```python
from build123d import *

# Parameters (mm, degrees)
SKETCH2_R                = 4
SKETCH2_R_2              = 3.5
BOSS_EXTRUDE1_DEPTH      = 10
BOSS_EXTRUDE2_REACH      = 15.601
BOSS_EXTRUDE2_END_RADIUS = 4
SKETCH3_R                = 3
SKETCH3_R_2              = 2.5
SKETCH4_R                = 4
BOSS_EXTRUDE3_DEPTH      = 0.5
FILLET2_R                = 0.5


with BuildPart() as part:
    # Sketch2 → Boss-Extrude1 (new body)
    with BuildSketch(Plane.XY.offset(8)):
        Circle(SKETCH2_R)
        Circle(SKETCH2_R_2, mode=Mode.SUBTRACT)
    extrude(amount=BOSS_EXTRUDE1_DEPTH)


with BuildPart() as body_2:
    # Mirror2: mirrored copy
    add(part.part.mirror(Plane.XY.offset(8)))

    # Boss-Extrude2: up to this cylinder (the profile starts outside it)
    boss_extrude2_end = Plane(origin=(0, 0, 5.872578), z_dir=(0, 0, 1)) * Cylinder(BOSS_EXTRUDE2_END_RADIUS, 40.202, mode=Mode.PRIVATE)
    # Sketch3 → Boss-Extrude2 (add, up to the surface)
    with BuildSketch(Plane(origin=(8, 0, 3), x_dir=(0, 0, -1), z_dir=(1, 0, 0)), mode=Mode.PRIVATE) as boss_extrude2_sk1:
        with Locations((0.042568871, 0)):
            Circle(SKETCH3_R)
        with Locations((0.042568871, 0)):
            Circle(SKETCH3_R_2, mode=Mode.SUBTRACT)
    boss_extrude2_tool1 = extrude(boss_extrude2_sk1.sketch, amount=-BOSS_EXTRUDE2_REACH, mode=Mode.PRIVATE) - boss_extrude2_end
    add(boss_extrude2_tool1.solids().sort_by_distance((8, 0, 5.872578))[0])

    # Sketch4 → Boss-Extrude3 (add)
    with BuildSketch(Plane(origin=(0, 0, -2), x_dir=(-1, 0, 0), z_dir=(0, 0, -1))):
        Circle(SKETCH4_R)
    extrude(amount=BOSS_EXTRUDE3_DEPTH)

    # Fillet2
    fillet2_edges = [body_2.edges().sort_by_distance(p)[0] for p in [
        (4, 0, -2.5),
    ]]
    fillet(fillet2_edges, radius=FILLET2_R - 0.0001)  # a hair under: the kernel refuses the full size


solid = body_2.part
```
Verification items for the finished model (mm, model axes). A direction names the side the tool comes from. Round coordinates to 2 decimals unless told otherwise and drop trailing zeros. Order: outer loops, then holes, each group sorted by start corner. A loop starts at its lowest first (then second) coordinate and runs counter-clockwise, first axis right, second up. Notation, with made-up numbers: (31, 11) -> (60, 11) arc R27 cw to (60, 30) -> close; hole circle Ø6 at (-28, 83.25). An arc over 180 degrees is marked (long way). Put each result on its own line as item: value. Start each with the question number.
(1) Section check D-D (x = 5.5). Enter the section's corners in (y, z), then the cut area to 3 significant figures.
(2) Draft check along Z on faces 4 (the face through (4, 0, 3)), 5 (the face through (8, 2, 1)), 6 (the face through (0, 0, -2)). Enter one of: +Z half, -Z half, draft (parallel to the pull), parting line (faces both ways), or undercut.
(3) Material ranges on line 1 along Y through (x, z) = (0, -0.5); line 2 along Z through (x, y) = (1, -1.25); line 3 along X through (y, z) = (2.5, 4.25), recorded low to high.
(4) Depth check by flat-ended pin: pin 1 Ø2 at (x, y) = (-1, -1) entering from +Z; pin 2 Ø3 at (y, z) = (-2.5, 0.5) entering from -X; pin 3 Ø1.5 at (x, z) = (2, 6) entering from -Y. Enter the tip coordinate at first touch or a pass-through.
(5) Section check C-C (z = 0.75). Enter the section's corners in (x, y), then the cut area to 3 significant figures.
(6) Section check B-B (y = 0). Enter the section's corners in (x, z), then the cut area to 3 significant figures.
(7) Tool access check on faces 1 (the face through (5.955, 0.132, 5.955)), 2 (the face through (0, 0, -2.5)), 3 (the face through (3.233, -1.341, 3.07)). Record the directions out of +Z, -Z, +X, -X, +Y, -Y that give a thin tool (end or side, any length) a straight path to the whole face; none if there is none.
(8) Section check A-A (x = 0). Enter the section's corners in (y, z).
Completed:
1. outline: circle Ø6 at (0, 2.96); hole circle Ø5 at (0, 2.96)
1. area: 8.64 mm2
2. face 4: undercut
2. face 5: draft
2. face 6: +Z half
3. line 1: y = -4 to -3.5, 3.5 to 4
3. line 2: z = -2.5 to -2
3. line 3: x = -3.12 to -2.45, 2.45 to 8
4. pin 1: stops at z = -2
4. pin 2: stops at x = -3.87
4. pin 3: stops at y = -3.8
5. outline: (3.45, -2.03) -> (8, -2.03) -> (8, -1.17) -> (3.82, -1.17) arc R4 ccw to (3.82, 1.17) -> (8, 1.17) -> (8, 2.03) -> (3.45, 2.03) arc R4 ccw (long way) to start; hole circle Ø7 at (0, 0)
5. area: 19.2 mm2
6. outline: (-4, -2) arc R0.5 ccw to (-3.5, -2.5) -> (3.5, -2.5) arc R0.5 ccw to (4, -2) -> (4, -0.04) -> (8, -0.04) -> (8, 0.46) -> (4, 0.46) -> (4, 5.46) -> (8, 5.46) -> (8, 5.96) -> (4, 5.96) -> (4, 8) -> (3.5, 8) -> (3.5, -2) -> (-3.5, -2) -> (-3.5, 8) -> (-4, 8) -> close
6. area: 17.9 mm2
7. face 1: +X
7. face 2: -Z, +X, -X, +Y, -Y
7. face 3: +Z
8. outline: (-4, -2) arc R0.5 ccw to (-3.5, -2.5) -> (3.5, -2.5) arc R0.5 ccw to (4, -2) -> (4, 8) -> (3.5, 8) -> (3.5, -2) -> (-3.5, -2) -> (-3.5, 8) -> (-4, 8) -> close
